from build123d import *

# Parameters (mm, degrees)
F0_W     = 101.6
F0_H     = 76.2
F0_R     = 12.7
F1_DEPTH = 12.7
F2_R     = 6.35
F3_DEPTH = 76.201
F4_R     = 5.08


with BuildPart() as f1:
    # F0 (on Front) → F1 (new body, symmetric)
    with BuildSketch(Plane.XZ):
        Rectangle(F0_W, F0_H)
        with Locations((6.35, 0)):
            Circle(F0_R, mode=Mode.SUBTRACT)
    extrude(amount=F1_DEPTH, both=True)

    # F2 (on face) → F3 (cut, through all)
    with BuildSketch(Plane.XY.offset(38.1)):
        with Locations((-25.4, 0)):
            Circle(F2_R)
    extrude(amount=-F3_DEPTH, mode=Mode.SUBTRACT)

    # F4
    f4_edges = [f1.edges().sort_by_distance(p)[0] for p in [
        (50.8, 0, 38.1),
        (-50.8, 0, 38.1),
        (50.8, 0, -38.1),
        (-50.8, 0, -38.1),
    ]]
    fillet(f4_edges, radius=F4_R)


solid = f1.part
Input: part model. Units: mm. Frame: model coordinates. Coordinates: 2 decimals unless noted, no trailing zeros. Loops run counter-clockwise (first coordinate to the right, second up) from the corner with the lowest first, then second, coordinate; pieces in that order, holes last.
Q1. Cut plane B-B (z = 0). Output: boundary loops of the cut face in (x, y).
Q2. Material intervals for line 1 (Z direction, x = 6.35, y = 3.75); line 2 (X direction, y = 9.5, z = 4); line 3 (X direction, y = 1.25, z = -21.5), sorted ascending.
Q3. Cut plane D-D (y = -10.75). Output: boundary loops of the cut face in (x, z), then the cut area to 3 significant figures.
Q4. Contact query for a flat-ended pin moving along its axis: pin 1 (23 mm diameter, centred on x = 6.35, z = 0, fed in from +Y). Output: stop coordinate, or through.
Q5. Cut plane C-C (x = 6.35). Output: boundary loops of the cut face in (y, z), then the cut area to 3 significant figures.
Q6. Draft query along X for faces 1 (the face through (-12, -12.7, 1)), 2 (the face through (-19.343, 1.907, 0.533)), 3 (the face through (-49.351, 0.178, 36.572)). Return one class per face: +X half, -X half, draft (parallel to the pull), parting line (faces both ways), or undercut.
Q7. Cut plane A-A (y = 0). Output: boundary loops of the cut face in (x, z).
Working result:
1. outline: (-50.8, -12.7) - (-6.35, -12.7) - (-6.35, 12.7) - (-50.8, 12.7) - close; (19.05, -12.7) - (50.8, -12.7) - (50.8, 12.7) - (19.05, 12.7) - close; hole circle Ø12.7 at (-25.4, 0)
2. line 1: z = -38.1 to -12.7, 12.7 to 38.1
2. line 2: x = -50.8 to -5.7, 18.4 to 50.8
2. line 3: x = -50.8 to -31.63, -19.17 to 50.8
3. outline: (-50.8, -33.02) arc R5.08 ccw to (-45.72, -38.1) - (45.72, -38.1) arc R5.08 ccw to (50.8, -33.02) - (50.8, 33.02) arc R5.08 ccw to (45.72, 38.1) - (-45.72, 38.1) arc R5.08 ccw to (-50.8, 33.02) - close; hole circle Ø25.4 at (6.35, 0)
3. area: 7,210 mm2
4. pin 1: passes through
5. outline: (-12.7, -38.1) - (12.7, -38.1) - (12.7, -12.7) - (-12.7, -12.7) - close; (-12.7, 12.7) - (12.7, 12.7) - (12.7, 38.1) - (-12.7, 38.1) - close
5. area: 1,290 mm2
6. face 1: draft
6. face 2: undercut
6. face 3: -X half
7. outline: (-50.8, -33.02) arc R5.08 ccw to (-45.72, -38.1) - (-31.75, -38.1) - (-31.75, 38.1) - (-45.72, 38.1) arc R5.08 ccw to (-50.8, 33.02) - close; (-19.05, -38.1) - (45.72, -38.1) arc R5.08 ccw to (50.8, -33.02) - (50.8, 33.02) arc R5.08 ccw to (45.72, 38.1) - (-19.05, 38.1) - close; hole circle Ø25.4 at (6.35, 0)
